```python
from build123d import *

# Parameters (mm, degrees)
SKETCH1_W                          = 35.56
SKETCH1_H                          = 146.05
EXTRUDE1_DEPTH                     = 1.5875
SKETCH3_W                          = 1.5875
SKETCH3_H                          = 103.886
EXTRUDE2_DEPTH                     = 9.398
F_32_0_116000_DIAMETER_HOLE1_D     = 2.9464
F_32_0_116000_DIAMETER_HOLE1_DEPTH = 25.4
F_32_0_116000_DIAMETER_HOLE1_TIP   = 0.885187864
SKETCH7_W                          = 35.56
SKETCH7_H                          = 1.5875
EXTRUDE3_DEPTH                     = 12.7


with BuildPart() as part:
    # Sketch1 → Extrude1 (new body)
    with BuildSketch(Plane.XY):
        with Locations((17.78, 73.025)):
            Rectangle(SKETCH1_W, SKETCH1_H)
    extrude(amount=EXTRUDE1_DEPTH)

    # Sketch3 → Extrude2 (add)
    with BuildSketch(Plane(origin=(35.56, 0, 0), x_dir=(0, 0, -1), z_dir=(1, 0, 0))):
        with Locations((-0.79375, 57.785)):
            Rectangle(SKETCH3_W, SKETCH3_H)
    extrude(amount=EXTRUDE2_DEPTH)

    # #32 (0.116000) Diameter Hole1
    with Locations(Plane(origin=(29.718, 9.779, 1.5875), x_dir=(1, 0, 0), z_dir=(0, 0, 1))):
        with Locations((0, 0), (0, 53.848), (0, 131.191)):
            Hole(F_32_0_116000_DIAMETER_HOLE1_D / 2, depth=F_32_0_116000_DIAMETER_HOLE1_DEPTH)
            with Locations((0, 0, -(F_32_0_116000_DIAMETER_HOLE1_DEPTH + F_32_0_116000_DIAMETER_HOLE1_TIP / 2))):  # 118° drill point
                Cone(0, F_32_0_116000_DIAMETER_HOLE1_D / 2, F_32_0_116000_DIAMETER_HOLE1_TIP, mode=Mode.SUBTRACT)

    # Sketch7 → Extrude3 (add)
    with BuildSketch(Plane(origin=(0, 146.05, 0), x_dir=(-1, 0, 0), z_dir=(0, 1, 0))):
        with Locations((-17.78, 0.79375)):
            Rectangle(SKETCH7_W, SKETCH7_H)
    extrude(amount=EXTRUDE3_DEPTH)


solid = part.part
```
Here's how the part is built. I have some questions about the finished solid (model axes, mm). Coordinates: 2 decimals unless noted, no trailing zeros. Loops run counter-clockwise (first coordinate to the right, second up) from the corner with the lowest first, then second, coordinate; pieces in that order, holes last. Notation, with made-up numbers: M 41.5,10.25 L 52.5,10.25 A19 ccw 52.5,23.25 Z; hole C -1.75,62.5 d5. An arc over 180 degrees is marked long. One line per item, written item: value.
1. Imagine slicing it at A-A (y = 140.97). List the corners of the cut face in (x, z) for me, and give its area (3 significant figures).
Geometry says:
outline: M 0,0 L 28.24,0 L 28.24,1.59 L 0,1.59 Z; M 31.19,0 L 35.56,0 L 35.56,1.59 L 31.19,1.59 Z
area: 51.8 mm2
2. Please list where these lines run through material, in increasing order: probe 1 along X at (y, z) = (147, 1.3); probe 2 along X at (y, z) = (140, 1.3); probe 3 along X at (y, z) = (9, 0.7).
Geometry says:
probe 1: x = 0 to 35.56
probe 2: x = 0 to 28.61, 30.83 to 35.56
probe 3: x = 0 to 28.47, 30.97 to 44.96
3. Imagine slicing it at C-C (x = 40). List the corners of the cut face in (y, z) for me, and give its area (3 significant figures).
Geometry says:
outline: M 5.84,0 L 109.73,0 L 109.73,1.59 L 5.84,1.59 Z
area: 165 mm2
4. Thinking about a two-plate mould opening in X: for faces 1 (the cylindrical face through (30.04, 62.19, 0.78)), 2 (the flat face through (23, 78, 1.588)), 3 (the cylindrical face through (29.91, 11.24, 0.78)), which applies, +X half, -X half, draft (parallel to the pull), parting line (faces both ways), or undercut?
Geometry says:
face 1: undercut
face 2: draft
face 3: undercut
5. Imagine slicing it at B-B (z = 1.15). List the corners of the cut face in (x, y) for me, and give its area (3 significant figures).
Geometry says:
outline: M 0,0 L 35.56,0 L 35.56,5.84 L 44.96,5.84 L 44.96,109.73 L 35.56,109.73 L 35.56,158.75 L 0,158.75 Z; hole C 29.72,9.78 d2.95; hole C 29.72,63.63 d2.95; hole C 29.72,140.97 d2.95
area: 6,600 mm2
6. Will these pins go through, and if not, where does the flat tip stop? pin 1 Ø1.8 at (x, y) = (29.718, 140.97) entering from +Z; pin 2 Ø0.5 at (y, z) = (2.5, 0.5) entering from +X.
Geometry says:
pin 1: passes through
pin 2: stops at x = 35.56
